Build history of the part. All positions in model axes, mm. Coordinates: 2 decimals unless noted, no trailing zeros. Write each loop counter-clockwise with the first axis right and the second up, starting at its lowest first coordinate (ties: lowest second). Pieces come first, ordered by that corner, then holes.
Autodesk Inventor part; units mm, degrees
ref_plane "MidSidePlane" through (0, 0, 10) normal (0, 0, 1) x (1, 0, 0)
ref_plane "YZ Plane" through (0, 0, 0) normal (1, 0, 0) x (0, 1, 0)
ref_plane "XZ Plane" through (0, 0, 0) normal (0, 1, 0) x (-1, 0, 0)
sketch "ShaftProfile" plane through (0, 0, 0) normal (0, 0, 1) x (1, 0, 0)
  line L0 (-56, 0) -> (70, 0) construction
  line L1 (-38, 9) -> (52, 9)
  line L2 (52, 9) -> (52, 0)
  line L3 (-38, 0) -> (-38, 9)
  line L4 (-38, 0) -> (52, 0)
  point P0 (0, 0)
  dimension "d1" = 90
  dimension "d2" = 9
  dimension "d4" = 38
revolve "ShaftFeature" add sketch "ShaftProfile" angle 360 about axis through (-38, 0, 0) along (1, 0, 0)
sketch "Sketch2" plane through (-38, 0, 0) normal (-1, 0, 0) x (0, 0, 1)
  circle A0 centre (0, 0) radius 9
hole "ShaftHoleFeature" at (-38, 0, 0) direction (1, 0, 0) diameter 16 end through all
ref_plane "MidSidePlane" through (0, 0, 10) normal (0, 0, 1) x (1, 0, 0)
sketch "CapHoles" plane through (0, 0, 10) normal (0, 0, 1) x (1, 0, 0)
  line L0 (52, -9) -> (52, 9) construction
  line L1 (-38, -9) -> (-38, 9) construction
  line L2 (-52, 0) -> (46, 0) construction
  circle A0 centre (-33.5, 0) radius 1.25
  circle A1 centre (47.5, 0) radius 1.25
  dimension "d24" = 2.5
  dimension "d25" = 4.5
  dimension "d26" = 4.5
extrude "CapHolesFeature" cut sketch "CapHoles" against normal through all
equation "\"d26\" = d25"
properties part number "BackPair1PistonShaft"
1. Saw through at A-A on z = 0. List the corners of the cut face in (x, y).
Computed values:
outline: (-38, -9) - (52, -9) - (52, -8) - (-38, -8) - close; (-38, 8) - (52, 8) - (52, 9) - (-38, 9) - close
2. Saw through at C-C on x = 21. List the corners of the cut face in (y, z).
Computed values:
outline: circle Ø18 at (0, 0); hole circle Ø16 at (0, 0)
3. Saw through at B-B on y = -6.25. List the corners of the cut face in (x, z), plus the area to 3 significant figures.
Computed values:
outline: (-38, -6.48) - (52, -6.48) - (52, -4.99) - (-38, -4.99) - close; (-38, 4.99) - (52, 4.99) - (52, 6.48) - (-38, 6.48) - close
area: 267 mm2
4. Flat gauge pins, fed straight in: pin 1 (1.5 mm diameter, centred on y = -5.5, z = -1.5, fed in from +X); pin 2 (1.5 mm diameter, centred on x = -8.5, y = -4, fed in from +Z); pin 3 (1 mm diameter, centred on x = -15, y = -5, fed in from -Z); pin 4 (2 mm diameter, centred on x = 30.5, y = -6, fed in from -Z). Where does each tip first touch, or does it go through?
Computed values:
pin 1: passes through
pin 2: stops at z = 8.39
pin 3: stops at z = -7.79
pin 4: stops at z = -7.48
5. Probe line 1 along X through (y, z) = (0, -8.5); line 2 along Z through (x, y) = (-9, 0); line 3 along Y through (x, z) = (-13, 6.25). List the from-to ranges inside material, lowest first.
Computed values:
line 1: x = -38 to -34.75, -32.25 to 46.25, 48.75 to 52
line 2: z = -9 to -8, 8 to 9
line 3: y = -6.48 to -4.99, 4.99 to 6.48
